Autodesk Inventor part; units mm, degrees
ref_plane "YZ Plane" through (0, 0, 0) normal (1, 0, 0) x (0, 1, 0)
ref_plane "XZ Plane" through (0, 0, 0) normal (0, 1, 0) x (-1, 0, 0)
ref_plane "XY Plane" through (0, 0, 0) normal (0, 0, 1) x (1, 0, 0)
sketch "Sketch1" plane through (0, 0, 0) normal (0, 0, 1) x (1, 0, 0)
  line L0 (0, 0) -> (0, 5.842)
  line L1 (0, 0) -> (5.842, 0) construction
  line L2 (0, 5.842) -> (-25.4, 5.842)
  line L3 (0, 5.842) -> (25.4, 5.842) construction
  line L4 (-25.4, 5.842) -> (-25.4, 2.667)
  line L5 (-25.4, 2.667) -> (-12.7, 2.667)
  line L6 (-25.4, 2.667) -> (-12.7, 2.667) construction
  line L7 (-12.7, 2.667) -> (-12.7, 0)
  line L8 (-12.7, 0) -> (0, 0)
  dimension "d0" = 5.842
  dimension "d1" = 90
  dimension "d2" = 25.4
  dimension "d3" = 180
  dimension "d4" = 3.175
  dimension "d5" = 12.7
  dimension "d6" = 0
extrude "Extrusion1" add sketch "Sketch1" along normal blind 25.4
properties part number "ToteBasinBracket"
Work out the finished part from the listing and answer in its coordinate system (mm). A direction names the side the tool comes from. Give positions to 0.01 mm unless a question says otherwise; leave off trailing zeros. Loops run counter-clockwise (first coordinate to the right, second up) from the corner with the lowest first, then second, coordinate; pieces in that order, holes last. Notation, with made-up numbers: (27.25, 61) -> (32.25, 61) arc R14 cw to (32.25, 87) -> close; hole circle Ø5 at (13, 40.25). An arc over 180 degrees is marked (long way). Use a Markdown table: item, result. Add a question column.
1) The part is cut by section C-C, the plane y = 0.4. Determine the outline of the cut face in (x, z).
2) Consider line 1 along X through (y, z) = (0.4, 3.75); line 2 along Y through (x, z) = (-17.25, 23). Determine where each line is inside the solid, lowest interval first.
3) Each of these flat-tipped pins is pushed along its axis until it touches: P1, Ø2, axis at x = -20, z = 12, coming from the -Y side; P2, Ø0.8, axis at y = 1, z = 9, coming from the -X side. Where does it stop, or does it pass through?
4) The part is cut by section B-B, the plane x = -19. Determine the outline of the cut face in (y, z).
5) Which of the six approach directions +Z, -Z, +X, -X, +Y, -Y give full straight-line access (tool end or side, diameter ignored) to faces 1 (the flat face through (-10, 4, 0)), 2 (the flat face through (-12.7, 1, 13))?
6) The part is cut by section A-A, the plane z = 7.5. Determine the outline of the cut face in (x, y), plus the area to 3 significant figures.
Reported:
| question | item | result |
|---|---|---|
| 1 | outline | (-12.7, 0) -> (0, 0) -> (0, 25.4) -> (-12.7, 25.4) -> close |
| 2 | line 1 | x = -12.7 to 0 |
| 2 | line 2 | y = 2.67 to 5.84 |
| 3 | P1 | stops at y = 2.67 |
| 3 | P2 | stops at x = -12.7 |
| 4 | outline | (2.67, 0) -> (5.84, 0) -> (5.84, 25.4) -> (2.67, 25.4) -> close |
| 5 | face 1 | -Z, +X, -X, +Y, -Y |
| 5 | face 2 | +Z, -Z, -X, -Y |
| 6 | outline | (-25.4, 2.67) -> (-12.7, 2.67) -> (-12.7, 0) -> (0, 0) -> (0, 5.84) -> (-25.4, 5.84) -> close |
| 6 | area | 115 mm^2 |
